Geometry: final body of the model. Coordinates: model frame, mm. Coordinates: 2 decimals unless noted, no trailing zeros. Order: outer loops, then holes, each group sorted by start corner. A loop starts at its lowest first (then second) coordinate and runs counter-clockwise, first axis right, second up. Notation, with made-up numbers: (7.25, 23) -> (15.25, 23) arc R23 ccw to (15.25, 59) -> close; hole circle Ø7 at (12, 0). An arc over 180 degrees is marked (long way). Answer in a Markdown table with one row per item. Add a question column.
1) Section query B-B on y = -30. Return the cut outline in (x, z).
2) Ray query, line 1 (Y direction, x = 17, z = 2.55); line 2 (Y direction, x = -16.5, z = 4.25); line 3 (X direction, y = -28.5, z = 3.65). Return the intervals inside material, ascending. Write a range as from..to.
3) Section query A-A on z = 2.3. Return the cut outline in (x, y).
4) Contact query for flat-ended pins moving along their axis: P1, Ø4, axis at x = 17, y = -30, coming from the -Z side; P2, Ø6.5, axis at x = -17, y = 30, coming from the +Z side. Output: stop coordinate, or through.
```python
from build123d import *

# Parameters (mm, degrees)
ESQUISSE1_W        = 45
ESQUISSE1_H        = 80
ESQUISSE1_R        = 2.5
BOSS_EXTRU_1_DEPTH = 5
CONG_1_R           = 5


with BuildPart() as part:
    # Esquisse1 → Boss.-Extru.1 (new body)
    with BuildSketch(Plane.XY):
        Rectangle(ESQUISSE1_W, ESQUISSE1_H)
        with Locations((-17, 30)):
            Circle(ESQUISSE1_R, mode=Mode.SUBTRACT)
        with Locations(Location((-17, -30, 0), (0, 0, 180))):
            Circle(ESQUISSE1_R, mode=Mode.SUBTRACT)
        with Locations((17, -30)):
            Circle(ESQUISSE1_R, mode=Mode.SUBTRACT)
        with Locations(Location((17, 30, 0), (0, 0, 180))):
            Circle(ESQUISSE1_R, mode=Mode.SUBTRACT)
    extrude(amount=BOSS_EXTRU_1_DEPTH)

    # Congé1
    cong_1_edges = [part.edges().sort_by_distance(p)[0] for p in [
        (22.5, -40, 2.5),
        (-22.5, -40, 2.5),
        (-22.5, 40, 2.5),
        (22.5, 40, 2.5),
    ]]
    fillet(cong_1_edges, radius=CONG_1_R)


solid = part.part
```
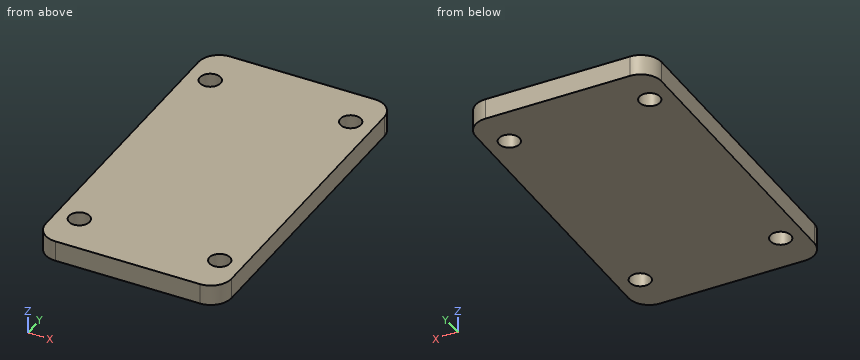
Result:
| question | item | result |
|---|---|---|
| 1 | outline | (-22.5, 0) -> (-19.5, 0) -> (-19.5, 5) -> (-22.5, 5) -> close; (-14.5, 0) -> (14.5, 0) -> (14.5, 5) -> (-14.5, 5) -> close; (19.5, 0) -> (22.5, 0) -> (22.5, 5) -> (19.5, 5) -> close |
| 2 | line 1 | -40..-32.5, -27.5..27.5, 32.5..40 |
| 2 | line 2 | -40..-32.45, -27.55..27.55, 32.45..40 |
| 2 | line 3 | -22.5..-19, -15..15, 19..22.5 |
| 3 | outline | (-22.5, -35) arc R5 ccw to (-17.5, -40) -> (17.5, -40) arc R5 ccw to (22.5, -35) -> (22.5, 35) arc R5 ccw to (17.5, 40) -> (-17.5, 40) arc R5 ccw to (-22.5, 35) -> close; hole circle Ø5 at (-17, -30); hole circle Ø5 at (-17, 30); hole circle Ø5 at (17, -30); hole circle Ø5 at (17, 30) |
| 4 | P1 | through |
| 4 | P2 | z = 5 |
